Check sheet for the modelled part. Datum: model origin and axes. Units: mm. Give positions to 0.01 mm unless a question says otherwise; leave off trailing zeros.
Item 1: Release check for a two-part mould opening along Y. For faces 1 (the cylindrical face through (9.08, 6.75, 3.91)), 2 (the flat face through (10, 0, 4)), 3 (the flat face through (0, 2, 4)), 4 (the cylindrical face through (15.12, 9.368, 7.485)) record: released by +Y, released by -Y, zero draft, split by the parting line, or undercut.
Item 2: Gauge pin test, flat ends, axial feed: P1, Ø3.5, axis at x = 9.52, y = 8.73, coming from the -Z side; P2, Ø1, axis at y = 1.5, z = 1, coming from the +X side; P3, Ø3, axis at x = 10.5, y = 8.5, coming from the +Z side. Record the tip position at first contact, or that the pin passes through.
Item 3: Material ranges on line 1 along Z through (x, y) = (4.5, 1.5); line 2 along X through (y, z) = (7.75, 6.75); line 3 along X through (y, z) = (0.75, 2.75), recorded low to high.
Item 4: Sectioned sample at A-A on z = 2.25. Count the separate pieces of the cut face and the enclosed holes in it, and give its area (3 significant figures).
from build123d import *

# Parameters (mm, degrees)
SKETCH1_R           = 2.032
BOSS_EXTRUDE1_DEPTH = 7.9375
SKETCH2_R           = 2.032
CUT_EXTRUDE1_DEPTH  = 25.6574065
FILLET1_R           = 1.5875


with BuildPart() as part:
    # Sketch1 → Boss-Extrude1 (new body)
    with BuildSketch(Plane.XY):
        with BuildLine():
            Line((0, 0), (0, 4.971229117))
            ThreePointArc((0, 4.971229117), (0.262744783, 6.235900833), (1.007492629, 7.291258599))
            Line((1.007492629, 7.291258599), (6.273738944, 12.211294223))
            ThreePointArc((6.273738944, 12.211294223), (9.525, 13.49375), (12.776261056, 12.211294223))
            Line((12.776261056, 12.211294223), (18.042507371, 7.291258599))
            ThreePointArc((18.042507371, 7.291258599), (18.787255217, 6.235900833), (19.05, 4.971229117))
            Line((19.05, 4.971229117), (19.05, 0))
            Line((19.05, 0), (0, 0))
        make_face()
        with Locations((9.525, 8.73125)):
            Circle(SKETCH1_R, mode=Mode.SUBTRACT)
    extrude(amount=BOSS_EXTRUDE1_DEPTH)

    # Sketch2 → Cut-Extrude1 (cut, through all)
    with BuildSketch(Plane.XZ):
        with Locations(Location((3.96875, 3.96875, 0), (0, 0, 270))):
            Circle(SKETCH2_R)
        with Locations(Location((15.08125, 3.96875, 0), (0, 0, 270))):
            Circle(SKETCH2_R)
    extrude(amount=-CUT_EXTRUDE1_DEPTH, mode=Mode.SUBTRACT)

    # Fillet1
    fillet1_edges = [part.edges().sort_by_distance(p)[0] for p in [
        (15.409384213, 9.751276411, 0),
        (18.787255217, 6.235900833, 0),
        (19.05, 2.485614558, 0),
        (18.787255217, 6.235900833, 7.9375),
        (15.409384213, 9.751276411, 7.9375),
        (9.525, 13.49375, 7.9375),
        (3.640615787, 9.751276411, 7.9375),
        (0.262744783, 6.235900833, 7.9375),
        (0, 2.485614558, 7.9375),
        (0, 2.485614558, 0),
        (19.05, 2.485614558, 7.9375),
        (0.262744783, 6.235900833, 0),
        (3.640615787, 9.751276411, 0),
        (9.525, 13.49375, 0),
    ]]
    fillet(fillet1_edges, radius=FILLET1_R)


solid = part.part
Report:
1. face 1: undercut
1. face 2: released by -Y
1. face 3: zero draft
1. face 4: released by +Y
2. P1: passes through
2. P2: stops at x = 19.05
2. P3: stops at z = 7.94
3. line 1: z = 0 to 2.01, 5.93 to 7.94
3. line 2: x = 1.57 to 7.75, 11.3 to 17.48
3. line 3: x = 0 to 2.34, 5.59 to 13.46, 16.71 to 19.05
4. separate pieces: 3
4. enclosed holes: 1
4. area: 145 mm2
